Autodesk Inventor part; units mm, degrees
ref_plane "YZ Plane" through (0, 0, 0) normal (1, 0, 0) x (0, 1, 0)
ref_plane "XZ Plane" through (0, 0, 0) normal (0, 1, 0) x (-1, 0, 0)
ref_plane "XY Plane" through (0, 0, 0) normal (0, 0, 1) x (1, 0, 0)
sketch "スケッチ1" plane through (0, 0, 0) normal (0, 1, 0) x (-1, 0, 0)
  line L0 (-5.0796, -45.5704) -> (-5.0796, 73.9296)
  line L1 (-5.0796, 73.9296) -> (-4.5796, 74.4296)
  line L2 (-4.5796, 74.4296) -> (24.4204, 74.4296)
  line L3 (24.4204, 74.4296) -> (24.9204, 73.9296)
  line L4 (24.9204, 73.9296) -> (24.9204, -45.5704)
  line L5 (24.9204, -45.5704) -> (-5.0796, -45.5704)
  line L6 (1.9204, -47.0704) -> (1.9204, -50.5704)
  line L7 (1.9204, -50.5704) -> (17.9204, -50.5704)
  line L8 (17.9204, -50.5704) -> (17.9204, -47.0704)
  line L9 (17.9204, -47.0704) -> (1.9204, -47.0704)
  line L10 (2.9204, -47.0704) -> (2.9204, -45.5704)
  line L11 (16.9204, -45.5704) -> (16.9204, -47.0704)
  line L12 (31.4204, 56.4296) -> (30.9204, 56.9296)
  line L13 (30.9204, 56.9296) -> (30.9204, 71.9296)
  line L14 (30.9204, 71.9296) -> (31.4204, 72.4296)
  line L15 (31.4204, 72.4296) -> (38.4204, 72.4296)
  line L16 (38.4204, 72.4296) -> (38.9204, 71.9296)
  line L17 (38.9204, 71.9296) -> (38.9204, 56.9296)
  line L18 (38.9204, 56.9296) -> (38.4204, 56.4296)
  line L19 (38.4204, 56.4296) -> (31.4204, 56.4296)
  line L20 (31.4204, 56.4296) -> (31.4204, 72.4296)
  line L21 (30.9204, 70.4296) -> (27.9204, 70.4296)
  line L22 (27.9204, 70.4296) -> (27.9204, 58.4296)
  line L23 (27.9204, 58.4296) -> (30.9204, 58.4296)
  line L24 (38.4204, 56.4296) -> (38.4204, 72.4296)
  line L25 (27.9204, 66.9296) -> (24.9204, 66.9296)
  line L26 (27.4204, 66.9296) -> (27.4204, 61.9296)
  line L27 (27.9204, 61.9296) -> (24.9204, 61.9296)
  line L28 (24.9204, 73.9296) -> (-5.0796, 73.9296)
  line L29 (-5.0796, 97.1797) -> (24.9204, 97.1797)
  line L30 (24.9204, 97.1797) -> (24.9204, 105.1797)
  line L31 (24.9204, 105.1797) -> (-5.0796, 105.1797)
  line L32 (-5.0796, 105.1797) -> (-5.0796, 97.1797)
  line L33 (24.9204, 99.1797) -> (27.9204, 99.1797)
  line L34 (27.2723, 99.1797) -> (27.2723, 103.1797)
  line L35 (27.9204, 103.1797) -> (24.9204, 103.1797)
  line L36 (27.9204, 105.6797) -> (27.9204, 96.6797)
  line L37 (27.9204, 96.6797) -> (28.4204, 96.1797)
  line L38 (28.4204, 96.1797) -> (32.4204, 96.1797)
  line L39 (32.4204, 96.1797) -> (32.9204, 96.6797)
  line L40 (32.9204, 96.6797) -> (32.9204, 105.6797)
  line L41 (32.9204, 105.6797) -> (32.4204, 106.1797)
  line L42 (32.4204, 106.1797) -> (28.4204, 106.1797)
  line L43 (28.4204, 106.1797) -> (27.9204, 105.6797)
  line L44 (28.4204, 106.1797) -> (28.4204, 96.1797)
  line L45 (32.4204, 96.1797) -> (32.4204, 106.1797)
  line L46 (2.4204, -50.5704) -> (2.4204, -47.0704)
  line L47 (-0.0796, -40.5704) -> (-0.0796, 74.4296)
  line L48 (19.9204, 74.4296) -> (19.9204, -40.5704)
  line L49 (19.9204, -40.5704) -> (9.9204, -46.3439)
  line L50 (9.9204, -46.3439) -> (-0.0796, -40.5704)
  line L51 (-0.0796, -40.5704) -> (19.9204, -40.5704)
  line L52 (17.4204, -47.0704) -> (17.4204, -50.5704)
  line L53 (9.9204, -56.5156) -> (9.9204, 78.76)
  line L54 (9.9204, 93.5864) -> (9.9204, 108.5157)
  line L55 (19.9204, 105.1797) -> (19.9204, 97.1797)
  line L56 (22.5096, 101.1797) -> (35.2156, 101.1797)
  line L57 (27.9204, 103.1797) -> (27.2723, 102.4797)
  line L58 (27.2723, 102.4797) -> (24.9204, 102.4797)
  line L59 (24.9204, 99.8797) -> (27.2723, 99.8797)
  line L60 (27.2723, 99.8797) -> (27.9204, 99.1797)
  line L61 (-0.0796, 97.1797) -> (-0.0796, 105.1797)
  line L62 (24.9204, 66.2296) -> (27.4204, 66.2296)
  line L63 (27.4204, 66.2296) -> (27.9204, 66.9296)
  line L64 (27.4204, 62.6296) -> (27.9204, 61.9296)
  line L65 (27.4204, 62.6296) -> (24.9204, 62.6296)
  line L66 (22.6428, 64.4296) -> (42.5049, 64.4296)
  line L67 (32.2954, 71.4296) -> (38.4204, 71.4296)
  line L68 (33.1704, 70.4296) -> (38.4204, 70.4296)
  line L69 (34.0454, 69.4296) -> (38.4204, 69.4296)
  line L70 (34.9204, 68.4296) -> (38.4204, 68.4296)
  line L71 (35.7954, 67.4296) -> (38.4204, 67.4296)
  line L72 (36.6704, 66.4296) -> (38.4204, 66.4296)
  line L73 (37.5454, 65.4296) -> (38.4204, 65.4296)
  line L74 (29.2204, 105.1797) -> (32.4204, 105.1797)
  line L75 (30.0204, 104.1797) -> (32.4204, 104.1797)
  line L76 (30.8204, 103.1797) -> (32.4204, 103.1797)
  line L77 (31.6204, 102.1797) -> (32.4204, 102.1797)
  point P0 (0, 0)
  point P1 (52.3578, -69.094)
  point P2 (52.3578, -59.2279)
  point P3 (24.9204, 64.4296)
  point P4 (38.9204, 64.4296)
revolve "回転1" add sketch "スケッチ1" angle 360 about axis through (-22.6428, 0, 64.4296) along (-1, 0, 0) contours L25 L26 L62 L4 | L62 L26 L66 L4 | L25 L63 L26 | L63 L22 L66 L26 | L22 L21 L13 L66 | L13 L14 L20 L66 | L20 L15 L24 L66 | L24 L16 L17 L66
thread "ねじ1"
properties part number "stand_handle" material "アルミニウム 6061"
For this review, take the finished solid that the model builds, in its own axes (mm). A direction names the side the tool comes from. Round coordinates to 2 decimals unless told otherwise and drop trailing zeros. Order: outer loops, then holes, each group sorted by start corner. A loop starts at its lowest first (then second) coordinate and runs counter-clockwise, first axis right, second up. Notation, with made-up numbers: (85, 44) -> (129, 44) arc R24 ccw to (129, 69) -> close; hole circle Ø6 at (87.25, 18.25). An arc over 180 degrees is marked (long way). Write item = value, one per line. Start each with the question number.
1) Take a section at A-A on y = 0. State the section outline as (x, z) points, plus the area to 4 significant figures.
2) To check wall thickness, follow line 1 (X direction, y = -4.25, z = 59.75); line 2 (X direction, y = 4, z = 60.25); line 3 (Y direction, x = -28.25, z = 64). State the ranges of each line that lie inside material, in increasing order. Write a range as from..to.
3) Insertion check: pin 1 (1.5 mm diameter, centred on x = -33.5, z = 65.5, fed in from +Y); pin 2 (5 mm diameter, centred on x = -28, y = -3.5, fed in from -Z); pin 3 (2 mm diameter, centred on y = 5.5, z = 66, fed in from +X). Each pin has a flat end and moves straight along its axis. Give the tip position at first contact, or say it passes through.
4) Tool access review of faces 1 (the face through (-30.92, 6, 67)), 2 (the face through (-24.92, 0, 64)): name each direction out of +Z, -Z, +X, -X, +Y, -Y from which nothing blocks a thin tool from reaching the whole face with its end or side.
5) Take a section at C-C on x = -30.25. State the section outline as (y, z) points.
6) Take a section at B-B on x = -33.5. State the section outline as (y, z) points, plus the area to 3 significant figures.
Verdict:
q1.outline = (-38.92, 56.93) -> (-38.42, 56.43) -> (-31.42, 56.43) -> (-30.92, 56.93) -> (-30.92, 58.43) -> (-27.92, 58.43) -> (-27.92, 61.93) -> (-24.92, 61.93) -> (-24.92, 66.93) -> (-27.92, 66.93) -> (-27.92, 70.43) -> (-30.92, 70.43) -> (-30.92, 71.93) -> (-31.42, 72.43) -> (-38.42, 72.43) -> (-38.92, 71.93) -> close
q1.area = 178.5 mm2
q2.line_1 = -38.92..-30.92
q2.line_2 = -38.92..-27.92
q2.line_3 = -5.98..5.98
q3.pin_1 = 7.99
q3.pin_2 = 58.51
q3.pin_3 = -27.92
q4.face_1 = +X
q4.face_2 = +Z, -Z, +X, +Y, -Y
q5.outline = circle Ø12 at (0, 64.43)
q6.outline = circle Ø16 at (0, 64.43)
q6.area = 201 mm2
